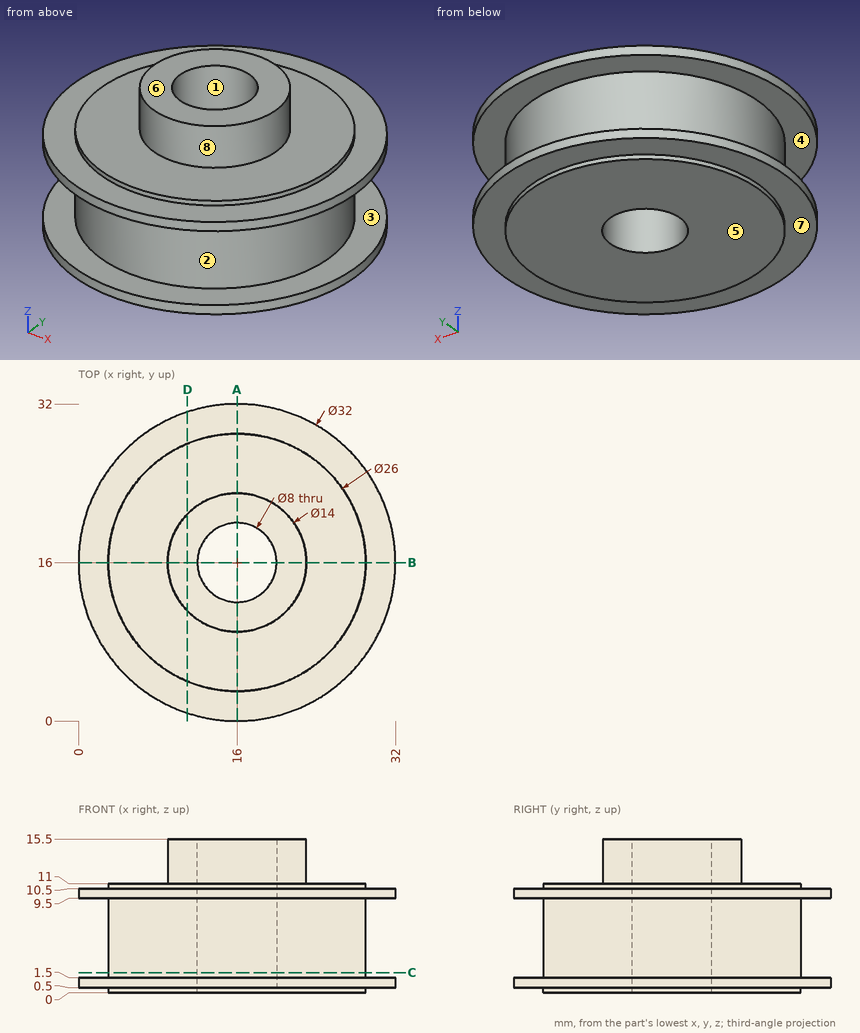
Verification items for this drawing (mm, ordinates from the low corner). A direction names the side the tool comes from. Give positions to 0.01 mm unless a question says otherwise; leave off trailing zeros. Write each loop counter-clockwise with the first axis right and the second up, starting at its lowest first coordinate (ties: lowest second). Pieces come first, ordered by that corner, then holes.
1) Go/stop test with flat-tipped pins: pin 1 Ø6 at (x, z) = (21.5, 2) entering from -Y; pin 2 Ø8 at (x, y) = (4.5, 11.5) entering from +Z; pin 3 Ø1.5 at (y, z) = (28.5, 2.5) entering from -X. Record where each tip stops, or that it passes through.
Values follow:
pin 1: stops at y = 0.2
pin 2: stops at z = 11
pin 3: stops at x = 10.44
2) Cross-section at A-A (x = 16). Record the boundary of the cut face in (y, z), plus the area to 3 significant figures.
Values follow:
outline: (0, 0.5) - (3, 0.5) - (3, 0) - (12, 0) - (12, 15.5) - (9, 15.5) - (9, 11) - (3, 11) - (3, 10.5) - (0, 10.5) - (0, 9.5) - (3, 9.5) - (3, 1.5) - (0, 1.5) - close; (20, 0) - (29, 0) - (29, 0.5) - (32, 0.5) - (32, 1.5) - (29, 1.5) - (29, 9.5) - (32, 9.5) - (32, 10.5) - (29, 10.5) - (29, 11) - (23, 11) - (23, 15.5) - (20, 15.5) - close
area: 237 mm2
3) Cross-section at C-C (z = 2). Record the boundary of the cut face in (x, y), plus the area to 3 significant figures.
Values follow:
outline: circle Ø26 at (16, 16); hole circle Ø8 at (16, 16)
area: 481 mm2
4) Release check for a two-part mould opening along X. For the marked faces 1, 2 and 3 record: released by +X, released by -X, zero draft, split by the parting line, or undercut.
Values follow:
face 1: undercut
face 2: split by the parting line
face 3: zero draft
5) Thickness scan on line 1 (Y direction, x = 16, z = 9); line 2 (Z direction, x = 29, y = 23); line 3 (Z direction, x = 7.5, y = 7). Record the ranges inside material, lowest first.
Values follow:
line 1: y = 3 to 12, 20 to 29
line 2: z = 0.5 to 1.5, 9.5 to 10.5
line 3: z = 0 to 11
6) Set-up check for the marked faces 4, 5, 6, 7 and 8: record each of +Z, -Z, +X, -X, +Y, -Y from which the full face is reachable in a straight line by a thin tool's end or side.
Values follow:
face 4: none
face 5: -Z, +X, -X, +Y, -Y
face 6: +Z, +X, -X, +Y, -Y
face 7: -Z
face 8: +Z
7) Cross-section at D-D (x = 11). Record the boundary of the cut face in (y, z), plus the area to 3 significant figures.
Values follow:
outline: (0.8, 0.5) - (4, 0.5) - (4, 0) - (28, 0) - (28, 0.5) - (31.2, 0.5) - (31.2, 1.5) - (28, 1.5) - (28, 9.5) - (31.2, 9.5) - (31.2, 10.5) - (28, 10.5) - (28, 11) - (20.9, 11) - (20.9, 15.5) - (11.1, 15.5) - (11.1, 11) - (4, 11) - (4, 10.5) - (0.8, 10.5) - (0.8, 9.5) - (4, 9.5) - (4, 1.5) - (0.8, 1.5) - close
area: 321 mm2
